CAD build for the part. Positions are in the model's coordinates, mm. Face numbers are marked on the shaded views. A direction names the side the tool comes from. Round coordinates to 2 decimals unless told otherwise and drop trailing zeros. Loops run counter-clockwise (first coordinate to the right, second up) from the corner with the lowest first, then second, coordinate; pieces in that order, holes last. Notation, with made-up numbers: (39, 22.25) - (82, 22.25) arc R12 ccw to (82, 45.25) - close; hole circle Ø11 at (3, 81.5). An arc over 180 degrees is marked (long way). One line per question, with ' | ' between items.
```python
from build123d import *

# Parameters (mm, degrees)
F1_DEPTH = 80
F2_DEPTH = 22
F5_DEPTH = 22
F7_R     = 10
F8_DEPTH = 15


with BuildPart() as f1:
    # F0 (on Right) → F1 (new body)
    with BuildSketch(Plane.YZ):
        Polygon((0, 30), (0, 0), (34.641016, 0), (17.320508, 30), align=None)
        Polygon((-34.641016, 0), (0, 0), (0, 30), (-17.320508, 30), align=None)
    extrude(amount=F1_DEPTH)

    # F0 (on Right) → F2 (join)
    with BuildSketch(Plane.YZ):
        Polygon((-17.320508, 30), (0, 30), (17.320508, 30), (0, 60), align=None)
    extrude(amount=F2_DEPTH)

    # F4 (on face) → F5 (join)
    with BuildSketch(Plane.YZ.offset(80)):
        Polygon((0, 60), (-17.320508, 30), (17.320508, 30), align=None)
    extrude(amount=-F5_DEPTH)

    # F7 (on Top) → F8 (join)
    with BuildSketch(Plane.XY):
        with BuildLine():
            Line((65, -55), (65, 55))
            ThreePointArc((65, 55), (40, 80), (15, 55))
            Line((15, 55), (15, -55))
            ThreePointArc((15, -55), (40, -80), (65, -55))
        make_face()
        with Locations((40, -55)):
            Circle(F7_R, mode=Mode.SUBTRACT)
        with Locations((40, 55)):
            Circle(F7_R, mode=Mode.SUBTRACT)
    extrude(amount=F8_DEPTH)


solid = f1.part
```
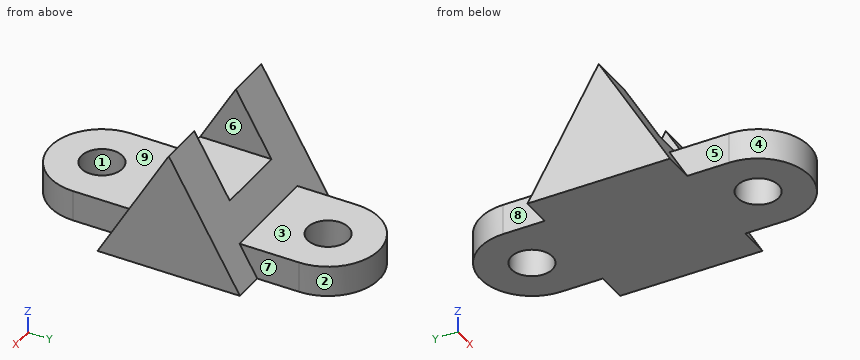
(1) Drop flat-ended pins along their axis: P1, Ø8, axis at x = 65.5, y = -59, coming from the +Z side; P2, Ø3, axis at x = 72, z = 12.5, coming from the +Y side; P3, Ø16.5, axis at y = 43, z = 9, coming from the -X side. Give the stop position or say it passes through.
Results found:
P1: stops at z = 15 | P2: stops at y = 28.29 | P3: stops at x = 15
(2) Cut at A-A, the plane x = 40. Write the cut outline in (y, z), then the cut area to 3 significant figures.
Results found:
outline: (-80, 0) - (-65, 0) - (-65, 15) - (-80, 15) - close; (-45, 0) - (45, 0) - (45, 15) - (25.98, 15) - (17.32, 30) - (-17.32, 30) - (-25.98, 15) - (-45, 15) - close; (65, 0) - (80, 0) - (80, 15) - (65, 15) - close | area: 2,450 mm²
(3) Probe L1, parallel to Y at x = 40, z = 3.75; L2, parallel to Z at x = 58, y = 71; L3, parallel to Z at x = 29.5, y = -4. List the from-to ranges inside material, lowest first.
Results found:
L1: y = -80 to -65, -45 to 45, 65 to 80 | L2: z = 0 to 15 | L3: z = 0 to 30
(4) Cut at B-B, the plane z = 55. Write the cut outline in (x, y), then the cut area to 3 significant figures.
Results found:
outline: (0, -2.89) - (22, -2.89) - (22, 2.89) - (0, 2.89) - close; (58, -2.89) - (80, -2.89) - (80, 2.89) - (58, 2.89) - close | area: 254 mm²
(5) Cut at D-D, the plane x = 25.5. Write the cut outline in (y, z), then the cut area to 3 significant figures.
Results found:
outline: (-75.37, 0) - (75.37, 0) - (75.37, 15) - (25.98, 15) - (17.32, 30) - (-17.32, 30) - (-25.98, 15) - (-75.37, 15) - close | area: 2,910 mm²
(6) Tool access for the marked faces 5, 6, 7, 8 and 9: list every direction of +Z, -Z, +X, -X, +Y, -Y with a clear straight run to the whole face (end or side of a thin tool).
Results found:
face 5: +Z, -X, -Y | face 6: +Z, +Y, -Y | face 7: +Z, +X, +Y | face 8: +Z, -X, +Y | face 9: +Z, +X, -X, -Y
(7) Cut at C-C, the plane y = 61.5. Write the cut outline in (x, z), then the cut area to 3 significant figures.
Results found:
outline: (15.86, 0) - (32.4, 0) - (32.4, 15) - (15.86, 15) - close; (47.6, 0) - (64.14, 0) - (64.14, 15) - (47.6, 15) - close | area: 496 mm²
(8) Two-plate mould, pull along Y, no slides. Class the marked faces 1, 2, 3 and 4: released by +Y, released by -Y, zero draft, split by the parting line, or undercut.
Results found:
face 1: undercut | face 2: released by +Y | face 3: zero draft | face 4: released by -Y
